```python
from build123d import *

# Parameters (mm, degrees)
SKETCH18_W                = 18
SKETCH18_H                = 26
SKETCH18_R                = 1.375
BOSS_EXTRUDE1_DEPTH       = 2.58
SKETCH19_W                = 1
SKETCH19_H                = 2.58
BOSS_EXTRUDE2_DEPTH       = 8
SKETCH20_W                = 26
SKETCH20_H                = 2.58
BOSS_EXTRUDE3_DEPTH       = 18
SKETCH21_R                = 1.375
CUT_EXTRUDE1_DEPTH        = 18
BOSS_EXTRUDE12_DEPTH      = 1
BOSS_EXTRUDE13_DEPTH      = 8
BOSS_EXTRUDE13_DEPTH_BACK = 1
SKETCH27_W                = 8
SKETCH27_H                = 1
BOSS_EXTRUDE14_DEPTH      = 2.5
SKETCH28_W                = 8
SKETCH28_H                = 1
BOSS_EXTRUDE15_DEPTH      = 2.5
BOSS_EXTRUDE16_DEPTH      = 1
BOSS_EXTRUDE17_DEPTH      = 9
SKETCH31_R                = 70
CUT_EXTRUDE8_DEPTH        = 17
SKETCH22_R                = 70
CUT_EXTRUDE9_DEPTH        = 17


with BuildPart() as part:
    # Sketch18 → Boss-Extrude1 (new body)
    with BuildSketch(Plane(origin=(0, 0, 0), x_dir=(1, 0, 0), z_dir=(0, 1, 0))):
        with Locations((9, 13)):
            Rectangle(SKETCH18_W, SKETCH18_H)
        with Locations(Location((9, 13, 0), (0, 0, 270))):
            Circle(SKETCH18_R, mode=Mode.SUBTRACT)
    extrude(amount=BOSS_EXTRUDE1_DEPTH)

    # Sketch19 → Boss-Extrude2 (add)
    with BuildSketch(Plane(origin=(18, 0, 0), x_dir=(0, 0, -1), z_dir=(1, 0, 0))):
        with Locations((0.5, 1.29)):
            Rectangle(SKETCH19_W, SKETCH19_H)
        with Locations((25.5, 1.29)):
            Rectangle(SKETCH19_W, SKETCH19_H)
    extrude(amount=BOSS_EXTRUDE2_DEPTH)

    # Sketch20 → Boss-Extrude3 (add)
    with BuildSketch(Plane(origin=(26, 0, 0), x_dir=(0, 0, -1), z_dir=(1, 0, 0))):
        with Locations((13, 1.29)):
            Rectangle(SKETCH20_W, SKETCH20_H)
    extrude(amount=BOSS_EXTRUDE3_DEPTH)

    # Sketch21 → Cut-Extrude1 (cut)
    with BuildSketch(Plane(origin=(0, 2.58, 0), x_dir=(1, 0, 0), z_dir=(0, 1, 0))):
        with Locations(Location((35, 13, 0), (0, 0, 270))):
            Circle(SKETCH21_R)
    extrude(amount=-CUT_EXTRUDE1_DEPTH, mode=Mode.SUBTRACT)

    # Sketch26_3 → Boss-Extrude13 (add, two sides: drawn at the far end of the back side and taken through both)
    with BuildSketch(Plane.ZY.offset(-26).offset(-BOSS_EXTRUDE13_DEPTH_BACK)):
        Polygon((13.62404816, -39.878327231), (-22.652991751, 0), (-24.00485771, 0), (12.884329852, -40.551243886), align=None)
        Polygon((4.34485947, -4.414818386), (3.605141162, -5.087735041), (25.459541086, -29.111660746), (26.199259394, -28.438744091), align=None)
        Polygon((-24.00485771, 0), (-22.652991751, 0), (-25, 2.58), (-25, 1.093931863), align=None)
    extrude(amount=BOSS_EXTRUDE13_DEPTH + BOSS_EXTRUDE13_DEPTH_BACK)


with BuildPart() as body_2:
    # Sketch26 → Boss-Extrude12 (new body)
    with BuildSketch(Plane.ZY.offset(-26)):
        Polygon((-1.0231364, 0), (-19.42564271, 0), (-21.280747396, 0), (-22.652991751, 0), (13.62404816, -39.878327231), (25.459541086, -29.111660746), (3.605141162, -5.087735041), align=None)
    extrude(amount=-BOSS_EXTRUDE12_DEPTH)



with BuildPart() as boss_extrude13_piece_1:
    # of the separate pieces the step leaves, piece 1, a body of its own (boss_extrude13_pieces)
    add(part.part.solids().sort_by_distance((0, 0, 0))[0])


with BuildPart() as boss_extrude13_piece_2:
    # of the separate pieces the step leaves, piece 2, a body of its own (boss_extrude13_pieces)
    add(part.part.solids().sort_by_distance((18, -5.087735041, 3.605141162))[0])


with BuildPart() as body_2_1:
    add(body_2.part)

    add(boss_extrude13_piece_2.part)  # Boss-Extrude14 merges Boss-Extrude13 piece 2
    # Sketch27 → Boss-Extrude14 (add)
    with BuildSketch(Plane(origin=(0, -0.509285347, -0.559843024), x_dir=(-1, 0, 0), z_dir=(0, -0.6729166552839775, -0.7397183078993143))):
        with Locations((-22, -38.16657766)):
            Rectangle(SKETCH27_W, SKETCH27_H)
    extrude(amount=BOSS_EXTRUDE14_DEPTH)


    add(boss_extrude13_piece_1.part)  # Boss-Extrude15 merges Boss-Extrude13 piece 1
    # Sketch28 → Boss-Extrude15 (add)
    with BuildSketch(Plane(origin=(0, -11.275951832, -12.39533595), x_dir=(1, 0, 0), z_dir=(0, 0.6729166552839719, 0.7397183078993194))):
        with Locations((22, -38.16657766)):
            Rectangle(SKETCH28_W, SKETCH28_H)
    extrude(amount=BOSS_EXTRUDE15_DEPTH)

    # Sketch29 → Boss-Extrude16 (add)
    with BuildSketch(Plane.ZY.offset(-18)):
        Polygon((-24.00485771, 0), (12.884329852, -40.551243886), (26.199259394, -28.438744091), (0.328729559, 0), align=None)
    extrude(amount=BOSS_EXTRUDE16_DEPTH)

    # Sketch32 → Boss-Extrude17 (add)
    with BuildSketch(Plane(origin=(18, 0, 0), x_dir=(0, 0, -1), z_dir=(1, 0, 0))):
        Polygon((-4.34485947, -4.414818386), (-3.605141162, -5.087735041), (1.0231364, 0), (-0.328729559, 0), align=None)
    extrude(amount=BOSS_EXTRUDE17_DEPTH)

    # Sketch31 → Cut-Extrude8 (cut)
    with BuildSketch(Plane.ZY.offset(-17)):
        with Locations((-13, -68.782265156)):
            Circle(SKETCH31_R)
    extrude(amount=CUT_EXTRUDE8_DEPTH, mode=Mode.SUBTRACT)

    # Sketch22 → Cut-Extrude9 (cut)
    with BuildSketch(Plane(origin=(44, 0, 0), x_dir=(0, 0, -1), z_dir=(1, 0, 0))):
        with Locations((13, -68.782265156)):
            Circle(SKETCH22_R)
    extrude(amount=-CUT_EXTRUDE9_DEPTH, mode=Mode.SUBTRACT)


solid = body_2_1.part
```
Design review of the part built by this model. Coordinates are the model's own, in mm. A direction names the side the tool comes from. Coordinates: 2 decimals unless noted, no trailing zeros. Loops run counter-clockwise (first coordinate to the right, second up) from the corner with the lowest first, then second, coordinate; pieces in that order, holes last. Notation, with made-up numbers: (-19.5, -21.75) -> (37.5, -21.75) arc R22 ccw to (37.5, 9.25) -> close; hole circle Ø7 at (86.25, 36.5). An arc over 180 degrees is marked (long way). Answer as a JSON object with one key per item and string values.
Q1. Clearance check with flat-ended pins moving along their axes: pin 1 Ø12.5 at (y, z) = (-14.5, -3.5) entering from +X; pin 2 Ø6 at (y, z) = (-23.5, 15.5) entering from -X; pin 3 Ø2.5 at (x, z) = (9, -13) entering from -Y; pin 4 Ø3 at (x, y) = (12.5, 1.5) entering from +Z. State where each tip first meets the part, or that it passes through.
Answer block:
{"pin 1": "stops at x = 27", "pin 2": "stops at x = 17", "pin 3": "passes through", "pin 4": "stops at z = 0"}
Q2. To check wall thickness, follow L1, parallel to X at y = 2, z = -13 (3 decimals); L2, parallel to X at y = -32.5, z = 21.5; L3, parallel to Z at x = 9, y = 2.25 (3 decimals). State the ranges of each line that lie inside material, in increasing order.
Answer block:
{"L1": "x = 0 to 7.625, 10.375 to 18, 26 to 33.625, 36.375 to 44", "L2": "x = 17 to 18, 26 to 27", "L3": "z = -26 to -14.375, -11.625 to 0"}
Q3. Take a section at C-C on y = -27.5. Give the boundary of the cut face in (x, z), plus the area to 3 significant figures.
Answer block:
{"outline": "(17, 1.01) -> (27, 1.01) -> (27, 25.35) -> (17, 25.35) -> close; hole (18, 2.36) -> (26, 2.36) -> (26, 23.99) -> (18, 23.99) -> close", "area": "70.3 mm^2"}
Q4. Take a section at B-B on z = -13. Give the boundary of the cut face in (x, y) (3 decimals).
Answer block:
{"outline": "(0, 1.218) -> (7.625, 1.218) -> (7.625, 2.58) -> (0, 2.58) -> close; (10.375, 1.218) -> (17, 1.218) -> (17, -12.097) -> (27, -12.097) -> (27, 1.218) -> (33.625, 1.218) -> (33.625, 2.58) -> (26, 2.58) -> (26, -10.611) -> (18, -10.611) -> (18, 2.58) -> (10.375, 2.58) -> close; (36.375, 1.218) -> (44, 1.218) -> (44, 2.58) -> (36.375, 2.58) -> close"}
Q5. Tool access review of faces 1 (the flat face through (22, 1, -1)), 2 (the flat face through (22, 1, 0)), 3 (the cylindrical face through (6.73, 1.217, -12.817)), 4 (the flat face through (22.056, -29.201, 23.875)), 5 (the flat face through (21.9, 0, -25.4)): name each direction out of +Z, -Z, +X, -X, +Y, -Y from which nothing blocks a thin tool from reaching the whole face with its end or side.
Answer block:
{"face 1": "+Y", "face 2": "+Z, +X, -X, +Y", "face 3": "-X, -Y", "face 4": "none", "face 5": "-Z, +X, -X, -Y"}
Q6. Take a section at A-A on x = 35. Give the boundary of the cut face in (y, z) (3 decimals), plus the area to 3 significant figures.
Answer block:
{"outline": "(0, -26) -> (2.58, -26) -> (2.58, -14.375) -> (1.204, -14.375) arc R70 cw to start; (0, 0) arc R70 cw to (1.204, -11.625) -> (2.58, -11.625) -> (2.58, 0) -> close", "area": "42.2 mm^2"}
Q7. The part is to be moulded in two halves that separate along X. For faces 6 (the flat face through (17, -15, 6)), 7 (the flat face through (17, 2.58, -13)), 8 (the flat face through (26, -18, 0)), say which applies: +X half, -X half, draft (parallel to the pull), parting line (faces both ways), or undercut.
Answer block:
{"face 6": "-X half", "face 7": "draft", "face 8": "undercut"}
